Design review of the part built by this model. Coordinates are the model's own, in mm. A direction names the side the tool comes from. Coordinates: 2 decimals unless noted, no trailing zeros. Loops run counter-clockwise (first coordinate to the right, second up) from the corner with the lowest first, then second, coordinate; pieces in that order, holes last. Notation, with made-up numbers: (-18.5, 37.25) - (39.5, 37.25) arc R36 cw to (39.5, 72.25) - close; hole circle Ø1 at (-29, 85.5). An arc over 180 degrees is marked (long way). Use one line per item in the form item = value. Start each with the question number.
(1) Add section C-C (y = -34). State the section outline as (x, z) points.
(2) Clearance check with flat-ended pins moving along their axes: pin 1 Ø3 at (x, y) = (0, 0) entering from +Z; pin 2 Ø1 at (x, z) = (1, 1.5) entering from +Y; pin 3 Ø3 at (x, y) = (1.5, -29) entering from -Z; pin 4 Ø2.5 at (x, y) = (0, -35) entering from -Z. State where each tip first meets the part, or that it passes through.
(3) Tool access review of faces 1 (the face through (0, -17, 2.5)), 2 (the face through (0, 0, 0.5)): name each direction out of +Z, -Z, +X, -X, +Y, -Y from which nothing blocks a thin tool from reaching the whole face with its end or side.
(4) For L1, parallel to Y at x = 0, z = 1.35; L2, parallel to Y at x = -1.25, z = 0.95; L3, parallel to X at y = 1, z = 2.2, list the stretches that pass through material, from the lowest coordinate up.
(5) Add section D-D (z = 1.25). State the section outline as (x, y) points, plus the area to 3 significant figures.
(6) Add section B-B (y = 1.5). State the section outline as (x, z) points, plus the area to 3 significant figures.
(7) The part is to be moulded in two halves that separate along Y. For faces 3 (the face through (0, -17, 0)), 4 (the face through (0, -39, 1)), 5 (the face through (1.847, 0.766, 1.232)), say which applies: pulls with the +Y half, pulls with the -Y half, needs draft (parallel to the pull), parting line crosses it, or undercut.
(8) Add section A-A (x = 0). State the section outline as (y, z) points.
Autodesk Inventor part; units mm, degrees
ref_plane "YZ Plane" through (0, 0, 0) normal (1, 0, 0) x (0, 1, 0)
ref_plane "XZ Plane" through (0, 0, 0) normal (0, 1, 0) x (-1, 0, 0)
ref_plane "XY Plane" through (0, 0, 0) normal (0, 0, 1) x (1, 0, 0)
sketch "Sketch1" plane through (0, 0, 0) normal (0, 0, 1) x (1, 0, 0)
  arc A0 (4, 0) -> (-4, 0) centre (0, 0) ccw
  arc A1 (-4, -35) -> (4, -35) centre (0, -35) ccw
  line L0 (0, 0) -> (0, -41.3039) construction
  line L1 (-4, 0) -> (-4, -35)
  line L2 (4, 0) -> (4, -35)
  circle A2 centre (0, 0) radius 2
  circle A3 centre (0, -35) radius 2
  dimension "d0" = 8
  dimension "d1" = 8
  dimension "d2" = 35
  dimension "d3" = 4
  dimension "d4" = 4
extrude "Extrusion1" add sketch "Sketch1" along normal blind 2.5
sketch "Sketch2" plane through (0, 0, 0) normal (1, 0, 0) x (0, 1, 0)
  line L0 (2, 2.5) -> (2, 0)
  line L1 (2, 1.25) -> (-2, 1.25)
  line L2 (-2, 2.5) -> (-2, 0)
  line L3 (2, 1.25) -> (-2, 1.25)
  line L4 (-2, 1.25) -> (-2, 2)
  line L5 (-2, 2) -> (2, 2)
  line L6 (2, 2) -> (2, 1.25)
  point P0 (0, 0)
  point P1 (2, 2)
  dimension "d7" = 1.5
revolve "Revolution1" add sketch "Sketch2" angle 360 about axis through (0, 2, 1.25) along (0, -1, 0)
properties part number "1-15"
Computed values:
q1.outline = (-4, 0) - (-1.73, 0) - (-1.73, 2.5) - (-4, 2.5) - close; (1.73, 0) - (4, 0) - (4, 2.5) - (1.73, 2.5) - close
q2.pin_1 = 2
q2.pin_2 = 3.97
q2.pin_3 = 0
q2.pin_4 = through
q3.face_1 = +Z, +X, -X, +Y, -Y
q3.face_2 = none
q4.L1 = -39 to -37, -33 to 4
q4.L2 = -38.8 to -36.56, -33.44 to -1.56, 1.56 to 3.8
q4.L3 = -3.87 to -1.73, 1.73 to 3.87
q5.outline = (-4, -35) arc R4 ccw to (4, -35) - (4, 0) arc R4 ccw to (-4, 0) - close; hole circle Ø4 at (0, -35); hole (-0.75, -1.85) - (-0.75, 1.85) arc R2 ccw to start; hole (0.75, -1.85) arc R2 ccw to (0.75, 1.85) - close
q5.area = 311 mm^2
q6.outline = (-3.71, 0) - (-1.32, 0) - (-1.32, 2.5) - (-3.71, 2.5) - close; circle Ø1.5 at (0, 1.25); (1.32, 0) - (3.71, 0) - (3.71, 2.5) - (1.32, 2.5) - close
q6.area = 13.7 mm^2
q7.face_3 = needs draft
q7.face_4 = pulls with the -Y half
q7.face_5 = undercut
q8.outline = (-39, 0) - (-37, 0) - (-37, 2.5) - (-39, 2.5) - close; (-33, 0) - (-2, 0) - (-2, 0.5) - (2, 0.5) - (2, 0) - (4, 0) - (4, 2.5) - (2, 2.5) - (2, 2) - (-2, 2) - (-2, 2.5) - (-33, 2.5) - close
